from build123d import *

# Parameters (mm, degrees)
SZKIC1_W                         = 22.5
SZKIC1_H                         = 12.2
DODANIE_WYCI_GNI_CIE1_DEPTH      = 22.2
DODANIE_WYCI_GNI_CIE2_DEPTH      = 4.6
DODANIE_WYCI_GNI_CIE2_DEPTH_BACK = 27.1
SZKIC2_W                         = 2.3
SZKIC2_H                         = 12.2
DODANIE_WYCI_GNI_CIE3_DEPTH      = 4.1
SZKIC8_R                         = 2.35
DODANIE_WYCI_GNI_CIE4_DEPTH      = 2.7
WYTNIJ_WYCI_GNI_CIE2_DEPTH       = 2.3
SZKIC11_R                        = 0.75
DODANIE_WYCI_GNI_CIE8_DEPTH      = 25.5


with BuildPart() as part:
    # Szkic1 → Dodanie-wyciągnięcie1 (new body)
    with BuildSketch(Plane.XY):
        with Locations((-11.470890411, -6.375490196)):
            Rectangle(SZKIC1_W, SZKIC1_H)
    extrude(amount=DODANIE_WYCI_GNI_CIE1_DEPTH)

    # Szkic2 → Dodanie-wyciągnięcie2 (add, two sides: drawn at the far end of the back side and taken through both)
    with BuildSketch(Plane(origin=(-0.220890411, 0, 0), x_dir=(0, 0, -1), z_dir=(1, 0, 0)).offset(-DODANIE_WYCI_GNI_CIE2_DEPTH_BACK)):
        with Locations((-17.05, -6.375490196)):
            Rectangle(SZKIC2_W, SZKIC2_H)
    extrude(amount=DODANIE_WYCI_GNI_CIE2_DEPTH + DODANIE_WYCI_GNI_CIE2_DEPTH_BACK)

    # Szkic3 → Dodanie-wyciągnięcie3 (add)
    with BuildSketch(Plane.XY.offset(22.2)):
        with BuildLine():
            Line((-10.770890411, -9.125490196), (-11.707558154, -9.125490196))
            ThreePointArc((-11.707558154, -9.125490196), (-22.720890411, -6.375490196), (-11.707558154, -3.625490196))
            Line((-11.707558154, -3.625490196), (-10.770890411, -3.625490196))
            ThreePointArc((-10.770890411, -3.625490196), (-8.020890411, -6.375490196), (-10.770890411, -9.125490196))
        make_face()
    extrude(amount=DODANIE_WYCI_GNI_CIE3_DEPTH)

    # Szkic8 → Dodanie-wyciągnięcie4 (add)
    with BuildSketch(Plane.XY.offset(26.3)):
        with Locations(Location((-16.870890411, -6.375490196, 0), (0, 0, 180))):
            Circle(SZKIC8_R)
    extrude(amount=DODANIE_WYCI_GNI_CIE4_DEPTH)

    # Szkic10 → Wytnij-wyciągnięcie2 (cut)
    with BuildSketch(Plane.XY.offset(18.2)):
        with BuildLine():
            Line((-27.320890411, -5.925490196), (-27.320890411, -6.925490196))
            Line((-27.320890411, -6.925490196), (-25.886915815, -6.925490196))
            ThreePointArc((-25.886915815, -6.925490196), (-24.020890411, -6.425490196), (-25.886915815, -5.925490196))
            Line((-25.886915815, -5.925490196), (-27.320890411, -5.925490196))
        make_face()
        with BuildLine():
            Line((4.379109589, -6.925490196), (2.945134993, -6.925490196))
            ThreePointArc((2.945134993, -6.925490196), (1.079109589, -6.425490196), (2.945134993, -5.925490196))
            Line((2.945134993, -5.925490196), (4.379109589, -5.925490196))
            Line((4.379109589, -5.925490196), (4.379109589, -6.925490196))
        make_face()
    extrude(amount=-WYTNIJ_WYCI_GNI_CIE2_DEPTH, mode=Mode.SUBTRACT)

    # Szkic11 → Dodanie-wyciągnięcie8 (add)
    with BuildSketch(Plane(origin=(-0.220890411, 0, 0), x_dir=(0, 0, -1), z_dir=(1, 0, 0))):
        with Locations((-4.45, -6.375490196)):
            Circle(SZKIC11_R)
        with Locations((-4.45, -4.825490196)):
            Circle(SZKIC11_R)
        with Locations((-4.45, -7.925490196)):
            Circle(SZKIC11_R)
    extrude(amount=-DODANIE_WYCI_GNI_CIE8_DEPTH)


solid = part.part
The listing builds one solid part. Answer for the finished solid, in the listing's coordinates (mm). A direction names the side the tool comes from. Round coordinates to 2 decimals unless told otherwise and drop trailing zeros. Write each loop counter-clockwise with the first axis right and the second up, starting at its lowest first coordinate (ties: lowest second). Pieces come first, ordered by that corner, then holes. Notation, with made-up numbers: (19, 24.5) - (52, 24.5) arc R18 ccw to (52, 44.5) - close; hole circle Ø3 at (-15, -24). An arc over 180 degrees is marked (long way). Use one line per item in the form item = value. Start each with the question number.
Item 1: Find the intervals of material crossed by line 1 (X direction, y = -11.5, z = 18.5); line 2 (Z direction, x = -10.5, y = -6.5); line 3 (Z direction, x = 3, y = -9.25), in increasing order. Write a range as [from, to].
Item 2: A tool of negligible diameter and unlimited length cuts with its end or side. For faces 5 (the flat face through (1, -6, 18.2)), 6 (the flat face through (-11, -3.625, 24)), 7 (the cylindrical face through (-24.2, -5.49, 4.1)), 8 (the cylindrical face through (-22.717, -6.593, 24.221)), 9 (the flat face through (4, -5.925, 17)), from which of +Z, -Z, +X, -X, +Y, -Y can it reach the whole face along a straight path? Write none if from no direction.
Item 3: A cutting plane is placed at C-C (x = -13). Write down the section's boundary in (y, z).
Item 4: A cutting plane is placed at A-A (z = 17). Write down the section's boundary in (x, y), plus the area to 3 significant figures.
Item 5: A cutting plane is placed at D-D (z = 4.45). Write down the section's boundary in (x, y).
Item 6: Flat-ended cylindrical pins translate along their axes: pin 1 Ø2.5 at (x, y) = (-26, -5) entering from -Z; pin 2 Ø4 at (x, y) = (-24, -4.5) entering from +Z; pin 3 Ø0.8 at (y, z) = (-4.5, 4) entering from -X. Find the tip coordinate at first contact, or state that the pin passes through.
Item 7: Determine the mould class of faces 1 (the flat face through (-25, -5, 15.9)), 2 (the cylindrical face through (-24.02, -6.46, 17.07)), 3 (the cylindrical face through (1.08, -6.46, 17.07)), 4 (the flat face through (-25.721, -8, 4)) for opening direction X: +X half, -X half, draft (parallel to the pull), parting line (faces both ways), or undercut.
Item 8: A cutting plane is placed at B-B (y = -2). Write down the section's boundary in (x, z).
The answers:
q1.line_1 = [-22.72, -0.22]
q1.line_2 = [0, 26.3]
q1.line_3 = [15.9, 18.2]
q2.face_5 = +Z, +X, +Y, -Y
q2.face_6 = +Z, +X, +Y
q2.face_7 = -X
q2.face_8 = +Z
q2.face_9 = +Z, -Z, +X
q3.outline = (-12.48, 0) - (-0.28, 0) - (-0.28, 22.2) - (-1.99, 22.2) - (-1.99, 26.3) - (-10.76, 26.3) - (-10.76, 22.2) - (-12.48, 22.2) - close
q4.outline = (-27.32, -12.48) - (4.38, -12.48) - (4.38, -6.93) - (2.95, -6.93) arc R1 cw (long way) to (2.95, -5.93) - (4.38, -5.93) - (4.38, -0.28) - (-27.32, -0.28) - (-27.32, -5.93) - (-25.89, -5.93) arc R1 cw (long way) to (-25.89, -6.93) - (-27.32, -6.93) - close
q4.area = 378 mm^2
q5.outline = (-25.72, -8.68) - (-22.72, -8.68) - (-22.72, -12.48) - (-0.22, -12.48) - (-0.22, -0.28) - (-22.72, -0.28) - (-22.72, -4.08) - (-25.72, -4.08) - (-25.72, -5.58) - (-22.72, -5.58) - (-22.72, -5.63) - (-25.72, -5.63) - (-25.72, -7.13) - (-22.72, -7.13) - (-22.72, -7.18) - (-25.72, -7.18) - close
q6.pin_1 = 3.7
q6.pin_2 = 26.3
q6.pin_3 = -25.72
q7.face_1 = draft
q7.face_2 = undercut
q7.face_3 = undercut
q7.face_4 = -X half
q8.outline = (-27.32, 15.9) - (-22.72, 15.9) - (-22.72, 0) - (-0.22, 0) - (-0.22, 15.9) - (4.38, 15.9) - (4.38, 18.2) - (-0.22, 18.2) - (-0.22, 22.2) - (-12.99, 22.2) - (-12.99, 26.3) - (-20.75, 26.3) - (-20.75, 22.2) - (-22.72, 22.2) - (-22.72, 18.2) - (-27.32, 18.2) - close
